```python
from build123d import *

# Parameters (mm, degrees)
SKETCH1_W               = 80
SKETCH1_H               = 36
BOSS_EXTRUDE1_DEPTH     = 1.6
SKETCH3_W               = 66
SKETCH3_H               = 16
BOSS_EXTRUDE2_DEPTH     = 3.9
SKETCH4_R               = 1.25
CUT_EXTRUDE1_DEPTH      = 4.9
MIRROR3_COPY_1_SKETCH_R = 1.25
MIRROR3_COPY_1_DEPTH    = 4.9


with BuildPart() as part:
    # Sketch1 → Boss-Extrude1 (new body)
    with BuildSketch(Plane(origin=(0, 0, 0), x_dir=(1, 0, 0), z_dir=(0, 1, 0))):
        Rectangle(SKETCH1_W, SKETCH1_H)
    extrude(amount=BOSS_EXTRUDE1_DEPTH)

    # Sketch3 → Boss-Extrude2 (add)
    with BuildSketch(Plane(origin=(0, 1.6, 0), x_dir=(1, 0, 0), z_dir=(0, 1, 0))):
        Rectangle(SKETCH3_W, SKETCH3_H)
    extrude(amount=BOSS_EXTRUDE2_DEPTH)

    # Sketch4 → Cut-Extrude1 (cut)
    with BuildSketch(Plane(origin=(0, 1.6, 0), x_dir=(1, 0, 0), z_dir=(0, 1, 0))):
        with Locations(Location((-37.5, 15.5, 0), (0, 0, 270))):
            Circle(SKETCH4_R)
    cut_extrude1 = extrude(amount=-CUT_EXTRUDE1_DEPTH, mode=Mode.SUBTRACT)

    # Mirror2: Cut-Extrude1 across plane
    add(cut_extrude1.mirror(Plane.ZY), mode=Mode.SUBTRACT)

    # Mirror3: Cut-Extrude1 across plane
    add(cut_extrude1.mirror(Plane.XY), mode=Mode.SUBTRACT)

    # Mirror3 copy 1 sketch → Mirror3 copy 1 (cut)
    with BuildSketch(Plane(origin=(0, 1.6, 0), x_dir=(-1, 0, 0), z_dir=(0, 1, 0))):
        with Locations(Location((-37.5, 15.5, 0), (0, 0, 270))):
            Circle(MIRROR3_COPY_1_SKETCH_R)
    extrude(amount=-MIRROR3_COPY_1_DEPTH, mode=Mode.SUBTRACT)


solid = part.part
```
Input: part model. Units: mm. Frame: model coordinates. A direction names the side the tool comes from. Coordinates: 2 decimals unless noted, no trailing zeros. Order: outer loops, then holes, each group sorted by start corner. A loop starts at its lowest first (then second) coordinate and runs counter-clockwise, first axis right, second up. Notation, with made-up numbers: (70.5, -33.75) - (120.5, -33.75) arc R17 ccw to (120.5, -26.75) - close; hole circle Ø1 at (25.5, -0.75). An arc over 180 degrees is marked (long way). Put each result on its own line as item: value.
1. Cut plane D-D on z = -4.5. Return the cut outline in (x, y), then the cut area to 3 significant figures.
Report:
outline: (-40, 0) - (40, 0) - (40, 1.6) - (33, 1.6) - (33, 5.5) - (-33, 5.5) - (-33, 1.6) - (-40, 1.6) - close
area: 385 mm2
2. Cut plane A-A on x = -37.5. Return the cut outline in (y, z).
Report:
outline: (0, -18) - (1.6, -18) - (1.6, -16.75) - (0, -16.75) - close; (0, -14.25) - (1.6, -14.25) - (1.6, 14.25) - (0, 14.25) - close; (0, 16.75) - (1.6, 16.75) - (1.6, 18) - (0, 18) - close
3. Reachability of faces 4 (the face through (0, 4, -8)), 5 (the face through (33, 4, 0)), 6 (the face through (-33, 4, 0)) from +Z, -Z, +X, -X, +Y, -Y: full face, straight path, thin tool, end or side. Return the list, or none.
Report:
face 4: -Z, +X, -X, +Y
face 5: +Z, -Z, +X, +Y
face 6: +Z, -Z, -X, +Y
4. Draft query along Z for faces 1 (the face through (-1, 1, -18)), 2 (the face through (40, 1, 0)), 3 (the face through (38.72, 0.81, -15.77)). Return one class per face: pulls with the +Z half, pulls with the -Z half, needs draft (parallel to the pull), parting line crosses it, or undercut.
Report:
face 1: pulls with the -Z half
face 2: needs draft
face 3: undercut
5. Line query: line 1 along Z through (x, y) = (37.5, 0.95); line 2 along X through (y, z) = (0.8, -15.5); line 3 along Z through (x, y) = (18, 2.35). Output: solid intervals per line, ascending.
Report:
line 1: z = -18 to -16.75, -14.25 to 14.25, 16.75 to 18
line 2: x = -40 to -38.75, -36.25 to 36.25, 38.75 to 40
line 3: z = -8 to 8
6. Cut plane C-C on x = 9.5. Return the cut outline in (y, z), then the cut area to 3 significant figures.
Report:
outline: (0, -18) - (1.6, -18) - (1.6, -8) - (5.5, -8) - (5.5, 8) - (1.6, 8) - (1.6, 18) - (0, 18) - close
area: 120 mm2
7. Cut plane B-B on z = -15.5. Return the cut outline in (x, y), then the cut area to 3 significant figures.
Report:
outline: (-40, 0) - (-38.75, 0) - (-38.75, 1.6) - (-40, 1.6) - close; (-36.25, 0) - (36.25, 0) - (36.25, 1.6) - (-36.25, 1.6) - close; (38.75, 0) - (40, 0) - (40, 1.6) - (38.75, 1.6) - close
area: 120 mm2
8. Contact query for flat-ended pins moving along their axis: pin 1 Ø1 at (x, z) = (5.5, -10) entering from +Y; pin 2 Ø1.2 at (x, y) = (-16, 3) entering from +Z; pin 3 Ø1.2 at (y, z) = (3.5, 3.5) entering from +X. Output: stop coordinate, or through.
Report:
pin 1: stops at y = 1.6
pin 2: stops at z = 8
pin 3: stops at x = 33
